Input: part model. Units: mm. Frame: model coordinates. A direction names the side the tool comes from. Coordinates: 2 decimals unless noted, no trailing zeros. Order: outer loops, then holes, each group sorted by start corner. A loop starts at its lowest first (then second) coordinate and runs counter-clockwise, first axis right, second up. Notation, with made-up numbers: (-27.75, -10) - (2.25, -10) arc R31 ccw to (2.25, 27) - close; hole circle Ø10 at (47, 23.25). An arc over 180 degrees is marked (long way). One line per question, with ' | ' between items.
from build123d import *

# Parameters (mm, degrees)
PAD_DEPTH       = 4.1
SKETCH002_R     = 1.5
SKETCH002_R_2   = 1.6
POCKET_DEPTH    = 16.101
SKETCH003_W     = 7
SKETCH003_H     = 6.2
POCKET001_DEPTH = 3
POCKET002_DEPTH = 16.101
POCKET003_DEPTH = 2


with BuildPart() as part:
    # Sketch → Pad (new body, symmetric)
    with BuildSketch(Plane.YZ):
        Polygon((-10.1, -9), (-10.1, 7), (6, 7), (6, 0), (3, 0), (3, -9), (0, -9), (0, 0), (-8.1, 0), (-8.1, -9), align=None)
    extrude(amount=PAD_DEPTH, both=True)

    # Sketch002 (on Face1 of Pad) → Pocket (cut, through all)
    with BuildSketch(Plane(origin=(0, -10.1, 0), x_dir=(0, 0, -1), z_dir=(0, -1, 0))):
        with Locations((-2.5, 0)):
            Circle(SKETCH002_R)
        with Locations((4.7, 0)):
            Circle(SKETCH002_R_2)
    extrude(amount=-POCKET_DEPTH, mode=Mode.SUBTRACT)

    # Sketch003 (on Face9 of Pocket) → Pocket001 (cut)
    with BuildSketch(Plane.ZX.offset(6)):
        with Locations((3.5, 0)):
            Rectangle(SKETCH003_W, SKETCH003_H)
    extrude(amount=-POCKET001_DEPTH, mode=Mode.SUBTRACT)

    # Sketch002 (on Face1 of Pad) → Pocket002 (cut, through all)
    with BuildSketch(Plane(origin=(0, -10.1, 0), x_dir=(0, 0, -1), z_dir=(0, -1, 0))):
        with Locations((-2.5, 0)):
            Circle(SKETCH002_R)
        with Locations((4.7, 0)):
            Circle(SKETCH002_R_2)
    extrude(amount=-POCKET002_DEPTH, mode=Mode.SUBTRACT)

    # Sketch004 (on Face19 of Pocket001) → Pocket003 (cut)
    with BuildSketch(Plane.ZX.offset(3)):
        Polygon((-7.875426, 0), (-6.287713, -2.75), (-3.112287, -2.75), (-1.524574, 0), (-3.112287, 2.75), (-6.287713, 2.75), align=None)
    extrude(amount=-POCKET003_DEPTH, mode=Mode.SUBTRACT)


solid = part.part
Item 1: Section C-C on z = -4.7. Return the cut outline in (x, y).
Data:
outline: (-4.1, -10.1) - (-1.6, -10.1) - (-1.6, -8.1) - (-4.1, -8.1) - close; (-4.1, 0) - (-1.6, 0) - (-1.6, 1) - (-2.75, 1) - (-2.75, 3) - (-4.1, 3) - close; (1.6, -10.1) - (4.1, -10.1) - (4.1, -8.1) - (1.6, -8.1) - close; (1.6, 0) - (4.1, 0) - (4.1, 3) - (2.75, 3) - (2.75, 1) - (1.6, 1) - close
Item 2: Section D-D on y = 4. Return the cut outline in (x, z).
Data:
outline: (-4.1, 0) - (-3.1, 0) - (-3.1, 7) - (-4.1, 7) - close; (3.1, 0) - (4.1, 0) - (4.1, 7) - (3.1, 7) - close
Item 3: Contact query for flat-ended pins moving along their axis: P1, Ø1, axis at x = -1, y = -1, coming from the -Z side; P2, Ø2.5, axis at x = 0, z = -4.7, coming from the +Y side; P3, Ø2.5, axis at x = 1.5, z = -2.5, coming from the +Y side. Output: stop coordinate, or through.
Data:
P1: z = 0 | P2: through | P3: y = 3
Item 4: Draft query along X for faces 1 (the face through (2, -8.1, -4)), 2 (the face through (-4.1, -2, 3)), 3 (the face through (0, -4, 1)). Return one class per face: released by +X, released by -X, zero draft, split by the parting line, or undercut.
Data:
face 1: zero draft | face 2: released by -X | face 3: undercut
Item 5: Section A-A on z = 2.5. Return the cut outline in (x, y).
Data:
outline: (-4.1, -10.1) - (-1.5, -10.1) - (-1.5, 3) - (-3.1, 3) - (-3.1, 6) - (-4.1, 6) - close; (1.5, -10.1) - (4.1, -10.1) - (4.1, 6) - (3.1, 6) - (3.1, 3) - (1.5, 3) - close
Item 6: Section B-B on y = -8.5. Return the cut outline in (x, z).
Data:
outline: (-4.1, -9) - (4.1, -9) - (4.1, 7) - (-4.1, 7) - close; hole circle Ø3.2 at (0, -4.7); hole circle Ø3 at (0, 2.5)
Item 7: Access query for faces 4 (the face through (3.6, 4.5, 0)), 5 (the face through (-1.394, 2.014, -2.33)), 6 (the face through (2, 0, -5)), 7 (the face through (-0.61, -9.11, -6.18)), 8 (the face through (3.1, 5, 3)). Directions: +Z, -Z, +X, -X, +Y, -Y. A direction counts if a zero-diameter tool reaches every point of the face in a straight line with its end or side. Return the directions, or none.
Data:
face 4: -Z, +X, -X, +Y | face 5: +Y | face 6: -Z, +X, -X | face 7: +Y, -Y | face 8: +Z, -Z, +Y
Item 8: Ray query, line 1 (X direction, y = 0.45, z = -4.7); line 2 (Y direction, x = 2, z = -5.25); line 3 (Y direction, x = -2.75, z = -2.75). Return the intervals inside material, ascending.
Data:
line 1: -4.1 to -1.6, 1.6 to 4.1 | line 2: -10.1 to -8.1, 0 to 1 | line 3: -10.1 to -8.1, 0 to 3
